Here's how the part is built. I have some questions about the finished solid (model axes, mm). A direction names the side the tool comes from. Round coordinates to 2 decimals unless told otherwise and drop trailing zeros. Order: outer loops, then holes, each group sorted by start corner. A loop starts at its lowest first (then second) coordinate and runs counter-clockwise, first axis right, second up. Notation, with made-up numbers: M -21,39.5 L -11,39.5 A21 cw -11,73.5 Z; hole C -37,-21 d6. An arc over 180 degrees is marked long. Write each question's results on one line, items separated by ' | '. Start each with the question number.
```python
from build123d import *

# Parameters (mm, degrees)
F0_R     = 12.065
F1_DEPTH = 42.7
F2_R     = 4.8
F3_DEPTH = 10
F4_W     = 6.5
F4_H     = 1.3
F5_DEPTH = 10
F6_R     = 10
F7_DEPTH = 25


with BuildPart() as f1:
    # F0 (on Top) → F1 (new body)
    with BuildSketch(Plane.XY):
        Circle(F0_R)
    extrude(amount=F1_DEPTH)

    # F2 (on face) → F3 (cut)
    with BuildSketch(Plane.XY.offset(42.7)):
        Circle(F2_R)
    extrude(amount=-F3_DEPTH, mode=Mode.SUBTRACT)

    # F4 (on face) → F5 (join)
    with BuildSketch(Plane.XY.offset(32.7)):
        Rectangle(F4_W, F4_H)
    extrude(amount=F5_DEPTH)

    # F6 (on face) → F7 (cut)
    with BuildSketch(Plane(origin=(0, 0, 0), x_dir=(1, 0, 0), z_dir=(0, 0, -1))):
        Circle(F6_R)
    extrude(amount=-F7_DEPTH, mode=Mode.SUBTRACT)


solid = f1.part
```
(1) I want a section at A-A on z = 40.5. Write out the boundary of the cut face in (x, y) (3 decimals).
(2) I want a section at D-D on z = 24.5. Write out the boundary of the cut face in (x, y) (3 decimals), and give its area (3 significant figures).
(3) Please list where these lines run through material, in increasing order: line 1 (Y direction, x = 0, z = 38.25) (3 decimals); line 2 (Z direction, x = -6, y = 2.5); line 3 (Z direction, x = -3.75, y = 0.5).
(4) I want a section at B-B on y = 0. Write out the boundary of the cut face in (x, z) (3 decimals), and give its area (3 significant figures).
(5) I want a section at C-C on x = -1. Write out the boundary of the cut face in (y, z).
(6) If we mould it in two halves opening along Y, with no side actions, what happens to faces 1 (the flat face through (0, -5, 42.7)), 2 (the cylindrical face through (11.51, 3.62, 21.05)), 3 (the cylindrical face through (-2.17, 9.76, 12.32))? For each: pulls with the +Y half, pulls with the -Y half, needs draft (parallel to the pull), parting line crosses it, or undercut.
(7) I'm going to push flat-ended pins straight in: pin 1 Ø12 at (x, y) = (-2.5, -1.5) entering from -Z; pin 2 Ø2 at (x, z) = (-1.5, 39.5) entering from +Y; pin 3 Ø12 at (y, z) = (8.5, 14) entering from -X. Where does each tip first touch, or does it pass through?
(8) On a 3-axis mill with a long thin cutter (end or side, diameter ignored), from which of +Z, -Z, +X, -X, +Y, -Y can I reach the whole of each face in a straight line? I mean faces 4 (the flat face through (-3.25, 0, 38)), 5 (the flat face through (-5, 9, 0)), 6 (the flat face through (0, 0, 25)). Say none if no direction works.
Solutions:
1) outline: C 0,0 d24.13; M -3.25,-0.65 L 3.25,-0.65 L 3.25,0.65 L -3.25,0.65 Z; hole C 0,0 d9.6
2) outline: C 0,0 d24.13; hole C 0,0 d20 | area: 143 mm^2
3) line 1: -12.065 to -4.8, -0.65 to 0.65, 4.8 to 12.065 | line 2: 25 to 42.7 | line 3: 25 to 32.7
4) outline: M -12.065,0 L -10,0 L -10,25 L 10,25 L 10,0 L 12.065,0 L 12.065,42.7 L 4.8,42.7 L 4.8,32.7 L 3.25,32.7 L 3.25,42.7 L -3.25,42.7 L -3.25,32.7 L -4.8,32.7 L -4.8,42.7 L -12.065,42.7 Z | area: 499 mm^2
5) outline: M -12.02,0 L -9.95,0 L -9.95,25 L 9.95,25 L 9.95,0 L 12.02,0 L 12.02,42.7 L 4.69,42.7 L 4.69,32.7 L 0.65,32.7 L 0.65,42.7 L -0.65,42.7 L -0.65,32.7 L -4.69,32.7 L -4.69,42.7 L -12.02,42.7 Z
6) face 1: needs draft | face 2: parting line crosses it | face 3: undercut
7) pin 1: z = 25 | pin 2: y = 12.05 | pin 3: x = -11.8
8) face 4: +Z | face 5: -Z, +X, -X, +Y, -Y | face 6: -Z
